The model under review builds one solid part; all positions refer to its coordinate system, in mm. Round coordinates to 2 decimals unless told otherwise and drop trailing zeros. Write each loop counter-clockwise with the first axis right and the second up, starting at its lowest first coordinate (ties: lowest second). Pieces come first, ordered by that corner, then holes. Notation, with made-up numbers: M 52,61.25 L 68,61.25 A35 ccw 68,96.25 Z; hole C 6.5,-38.5 d9. An arc over 180 degrees is marked long. Write item = value, one per line. Start each with the question number.
Item 1: Take a section at C-C, the plane z = -91. Give the boundary of the cut face in (x, y), plus the area to 3 significant figures.
Item 2: For pin 1 Ø1 at (y, z) = (15, -35) entering from -X; pin 2 Ø3 at (x, z) = (105.5, -212.5) entering from +Y; pin 3 Ø5 at (x, z) = (221.5, -97.5) entering from +Y, all flat-tipped, find the tip position at first contact; note any pin that passes through.
Item 3: To check wall thickness, follow line 1 along X through (y, z) = (2.25, -290); line 2 along Z through (x, y) = (260, 0.6); line 3 along X through (y, z) = (2.1, -190). State the ranges of each line that lie inside material, in increasing order.
Item 4: Take a section at A-A, the plane y = 23.5. Give the boundary of the cut face in (x, z), plus the area to 3 significant figures.
Item 5: Take a section at B-B, the plane x = 82. Give the boundary of the cut face in (y, z), plus the area to 3 significant figures.
from build123d import *

# Parameters (mm, degrees)
SKETCH1_W            = 270
SKETCH1_H            = 300
SKETCH1_R            = 2
BOSS_EXTRUDE1_DEPTH  = 3
SKETCH2_R            = 1.35
BOSS_EXTRUDE2_DEPTH  = 10
SKETCH3_R            = 2
BOSS_EXTRUDE3_DEPTH  = 15
SKETCH4_R            = 1.35
BOSS_EXTRUDE4_DEPTH  = 5
SKETCH5_R            = 2
BOSS_EXTRUDE5_DEPTH  = 15
SKETCH6_R            = 1.6
BOSS_EXTRUDE6_DEPTH  = 15
SKETCH7_R            = 2
BOSS_EXTRUDE7_DEPTH  = 15
CUT_EXTRUDE1_START   = -15
SKETCH8_R            = 1.6
CUT_EXTRUDE1_DEPTH   = 15
SKETCH9_R            = 1.6
BOSS_EXTRUDE8_DEPTH  = 15
CUT_EXTRUDE3_START   = -15
SKETCH10_R           = 1.6
CUT_EXTRUDE3_DEPTH   = 15
SKETCH11_R           = 1.6
BOSS_EXTRUDE9_DEPTH  = 15
SKETCH12_R           = 1.6
BOSS_EXTRUDE10_DEPTH = 15
CUT_EXTRUDE4_START   = -15
SKETCH13_R           = 2
CUT_EXTRUDE4_DEPTH   = 15
SKETCH14_R           = 1.35
BOSS_EXTRUDE11_DEPTH = 15
CUT_EXTRUDE7_START   = -15
SKETCH15_R           = 1.35
CUT_EXTRUDE7_DEPTH   = 15
SKETCH16_R           = 1.35
BOSS_EXTRUDE12_DEPTH = 15
SKETCH18_R           = 1.35
CUT_EXTRUDE9_DEPTH   = 15


with BuildPart() as part:
    # Sketch1 → Boss-Extrude1 (new body)
    with BuildSketch(Plane(origin=(0, 0, 0), x_dir=(1, 0, 0), z_dir=(0, 1, 0))):
        with Locations((135, 150)):
            Rectangle(SKETCH1_W, SKETCH1_H)
        with Locations(Location((10, 290, 0), (0, 0, 270))):
            Circle(SKETCH1_R, mode=Mode.SUBTRACT)
        with Locations(Location((10, 190, 0), (0, 0, 270))):
            Circle(SKETCH1_R, mode=Mode.SUBTRACT)
        with Locations(Location((10, 10, 0), (0, 0, 270))):
            Circle(SKETCH1_R, mode=Mode.SUBTRACT)
        with Locations(Location((135, 10, 0), (0, 0, 270))):
            Circle(SKETCH1_R, mode=Mode.SUBTRACT)
        with Locations(Location((260, 290, 0), (0, 0, 90))):
            Circle(SKETCH1_R, mode=Mode.SUBTRACT)
        with Locations(Location((260, 190, 0), (0, 0, 90))):
            Circle(SKETCH1_R, mode=Mode.SUBTRACT)
        with Locations(Location((260, 10, 0), (0, 0, 90))):
            Circle(SKETCH1_R, mode=Mode.SUBTRACT)
        with Locations(Location((135, 290, 0), (0, 0, 270))):
            Circle(SKETCH1_R, mode=Mode.SUBTRACT)
    extrude(amount=BOSS_EXTRUDE1_DEPTH)

    # Sketch2 → Boss-Extrude2 (add)
    with BuildSketch(Plane(origin=(0, 3, 0), x_dir=(1, 0, 0), z_dir=(0, 1, 0))):
        with Locations(Location((106, 270, 0), (0, 0, 90))):
            Circle(SKETCH2_R)
        with Locations(Location((155, 270, 0), (0, 0, 90))):
            Circle(SKETCH2_R)
        with Locations(Location((106, 212, 0), (0, 0, 90))):
            Circle(SKETCH2_R)
        with Locations(Location((155, 212, 0), (0, 0, 90))):
            Circle(SKETCH2_R)
    extrude(amount=BOSS_EXTRUDE2_DEPTH)

    # Sketch3 → Boss-Extrude3 (add)
    with BuildSketch(Plane(origin=(0, 3, 0), x_dir=(1, 0, 0), z_dir=(0, 1, 0))):
        with Locations(Location((150, 172.75, 0), (0, 0, 90))):
            Circle(SKETCH3_R)
        with Locations(Location((150, 127.25, 0), (0, 0, 90))):
            Circle(SKETCH3_R)
    extrude(amount=BOSS_EXTRUDE3_DEPTH)

    # Sketch4 → Boss-Extrude4 (add)
    with BuildSketch(Plane(origin=(0, 13, 0), x_dir=(1, 0, 0), z_dir=(0, 1, 0))):
        with Locations(Location((106, 212, 0), (0, 0, 90))):
            Circle(SKETCH4_R)
        with Locations(Location((155, 212, 0), (0, 0, 90))):
            Circle(SKETCH4_R)
        with Locations(Location((155, 270, 0), (0, 0, 90))):
            Circle(SKETCH4_R)
        with Locations(Location((106, 270, 0), (0, 0, 90))):
            Circle(SKETCH4_R)
    extrude(amount=BOSS_EXTRUDE4_DEPTH)

    # Sketch5 → Boss-Extrude5 (add)
    with BuildSketch(Plane(origin=(0, 3, 0), x_dir=(1, 0, 0), z_dir=(0, 1, 0))):
        with Locations(Location((41, 270, 0), (0, 0, 90))):
            Circle(SKETCH5_R)
        with Locations(Location((71, 270, 0), (0, 0, 90))):
            Circle(SKETCH5_R)
    extrude(amount=BOSS_EXTRUDE5_DEPTH)

    # Sketch6 → Boss-Extrude6 (add)
    with BuildSketch(Plane(origin=(0, 3, 0), x_dir=(1, 0, 0), z_dir=(0, 1, 0))):
        with Locations(Location((65, 75.462075724, 0), (0, 0, 90))):
            Circle(SKETCH6_R)
        with Locations(Location((105, 75.462075724, 0), (0, 0, 90))):
            Circle(SKETCH6_R)
        with Locations(Location((65, 35.462075724, 0), (0, 0, 90))):
            Circle(SKETCH6_R)
        with Locations(Location((105, 35.462075724, 0), (0, 0, 90))):
            Circle(SKETCH6_R)
        with Locations(Location((165, 35.462075724, 0), (0, 0, 90))):
            Circle(SKETCH6_R)
        with Locations(Location((205, 35.462075724, 0), (0, 0, 90))):
            Circle(SKETCH6_R)
        with Locations(Location((205, 75.462075724, 0), (0, 0, 90))):
            Circle(SKETCH6_R)
        with Locations(Location((165, 75.462075724, 0), (0, 0, 90))):
            Circle(SKETCH6_R)
    extrude(amount=BOSS_EXTRUDE6_DEPTH)

    # Sketch7 → Boss-Extrude7 (add)
    with BuildSketch(Plane(origin=(0, 3, 0), x_dir=(1, 0, 0), z_dir=(0, 1, 0))):
        with Locations(Location((41, 230, 0), (0, 0, 90))):
            Circle(SKETCH7_R)
        with Locations(Location((71, 230, 0), (0, 0, 90))):
            Circle(SKETCH7_R)
    extrude(amount=BOSS_EXTRUDE7_DEPTH)

    # Sketch8 → Cut-Extrude1 (cut)
    with BuildSketch(Plane(origin=(0, 18, 0), x_dir=(1, 0, 0), z_dir=(0, 1, 0)).offset(CUT_EXTRUDE1_START)):
        with Locations((205, 75.462075724)):
            Circle(SKETCH8_R)
        with Locations((205, 35.462075724)):
            Circle(SKETCH8_R)
    extrude(amount=CUT_EXTRUDE1_DEPTH, mode=Mode.SUBTRACT)

    # Sketch9 → Boss-Extrude8 (add)
    with BuildSketch(Plane(origin=(0, 3, 0), x_dir=(1, 0, 0), z_dir=(0, 1, 0))):
        with Locations(Location((185, 75.462075724, 0), (0, 0, 90))):
            Circle(SKETCH9_R)
        with Locations(Location((185, 35.462075724, 0), (0, 0, 90))):
            Circle(SKETCH9_R)
    extrude(amount=BOSS_EXTRUDE8_DEPTH)

    # Sketch10 → Cut-Extrude3 (cut)
    with BuildSketch(Plane(origin=(0, 18, 0), x_dir=(1, 0, 0), z_dir=(0, 1, 0)).offset(CUT_EXTRUDE3_START)):
        with Locations((185, 75.462075724)):
            Circle(SKETCH10_R)
        with Locations((185, 35.462075724)):
            Circle(SKETCH10_R)
    extrude(amount=CUT_EXTRUDE3_DEPTH, mode=Mode.SUBTRACT)

    # Sketch11 → Boss-Extrude9 (add)
    with BuildSketch(Plane(origin=(0, 18, 0), x_dir=(1, 0, 0), z_dir=(0, 1, 0))):
        with Locations(Location((205, 75.462075724, 0), (0, 0, 270))):
            Circle(SKETCH11_R)
        with Locations(Location((205, 35.462075724, 0), (0, 0, 270))):
            Circle(SKETCH11_R)
    extrude(amount=-BOSS_EXTRUDE9_DEPTH)

    # Sketch12 → Boss-Extrude10 (add)
    with BuildSketch(Plane(origin=(0, 18, 0), x_dir=(1, 0, 0), z_dir=(0, 1, 0))):
        with Locations(Location((65, 35.462075724, 0), (0, 0, 90))):
            Circle(SKETCH12_R)
        with Locations(Location((105, 35.462075724, 0), (0, 0, 90))):
            Circle(SKETCH12_R)
        with Locations(Location((105, 75.462075724, 0), (0, 0, 90))):
            Circle(SKETCH12_R)
        with Locations(Location((65, 75.462075724, 0), (0, 0, 90))):
            Circle(SKETCH12_R)
        with Locations(Location((165, 75.462075724, 0), (0, 0, 90))):
            Circle(SKETCH12_R)
        with Locations(Location((165, 35.462075724, 0), (0, 0, 90))):
            Circle(SKETCH12_R)
        with Locations(Location((205, 35.462075724, 0), (0, 0, 270))):
            Circle(SKETCH12_R)
        with Locations(Location((205, 75.462075724, 0), (0, 0, 270))):
            Circle(SKETCH12_R)
    extrude(amount=BOSS_EXTRUDE10_DEPTH)

    # Sketch13 → Cut-Extrude4 (cut)
    with BuildSketch(Plane(origin=(0, 18, 0), x_dir=(1, 0, 0), z_dir=(0, 1, 0)).offset(CUT_EXTRUDE4_START)):
        with Locations((41, 270)):
            Circle(SKETCH13_R)
        with Locations((41, 230)):
            Circle(SKETCH13_R)
    extrude(amount=CUT_EXTRUDE4_DEPTH, mode=Mode.SUBTRACT)

    # Sketch14 → Boss-Extrude11 (add)
    with BuildSketch(Plane(origin=(0, 18, 0), x_dir=(1, 0, 0), z_dir=(0, 1, 0))):
        with Locations(Location((155, 190, 0), (0, 0, 270))):
            Circle(SKETCH14_R)
        with Locations(Location((106, 190, 0), (0, 0, 270))):
            Circle(SKETCH14_R)
        with Locations(Location((106, 248, 0), (0, 0, 270))):
            Circle(SKETCH14_R)
        with Locations(Location((155, 248, 0), (0, 0, 90))):
            Circle(SKETCH14_R)
    extrude(amount=-BOSS_EXTRUDE11_DEPTH)

    # Sketch15 → Cut-Extrude7 (cut)
    with BuildSketch(Plane(origin=(0, 18, 0), x_dir=(1, 0, 0), z_dir=(0, 1, 0)).offset(CUT_EXTRUDE7_START)):
        with Locations((106, 212)):
            Circle(SKETCH15_R)
        with Locations((155, 212)):
            Circle(SKETCH15_R)
        with Locations((155, 270)):
            Circle(SKETCH15_R)
        with Locations((106, 270)):
            Circle(SKETCH15_R)
    extrude(amount=CUT_EXTRUDE7_DEPTH, mode=Mode.SUBTRACT)

    # Sketch16 → Boss-Extrude12 (add)
    with BuildSketch(Plane(origin=(0, 18, 0), x_dir=(1, 0, 0), z_dir=(0, 1, 0))):
        with Locations(Location((106, 270, 0), (0, 0, 270))):
            Circle(SKETCH16_R)
        with Locations(Location((155, 270, 0), (0, 0, 270))):
            Circle(SKETCH16_R)
        with Locations(Location((106, 212, 0), (0, 0, 270))):
            Circle(SKETCH16_R)
        with Locations(Location((155, 212, 0), (0, 0, 270))):
            Circle(SKETCH16_R)
    extrude(amount=-BOSS_EXTRUDE12_DEPTH)

    # Sketch18 → Cut-Extrude9 (cut)
    with BuildSketch(Plane(origin=(0, 18, 0), x_dir=(1, 0, 0), z_dir=(0, 1, 0))):
        with Locations((106, 248)):
            Circle(SKETCH18_R)
        with Locations((155, 248)):
            Circle(SKETCH18_R)
        with Locations((155, 190)):
            Circle(SKETCH18_R)
        with Locations((106, 190)):
            Circle(SKETCH18_R)
    extrude(amount=-CUT_EXTRUDE9_DEPTH, mode=Mode.SUBTRACT)


solid = part.part
Response values:
q1.outline = M 0,0 L 270,0 L 270,3 L 0,3 Z
q1.area = 810 mm2
q2.pin_1 = 63.4
q2.pin_2 = 18
q2.pin_3 = 3
q3.line_1 = 0 to 8, 12 to 133, 137 to 258, 262 to 270
q3.line_2 = -300 to -292, -288 to -192, -188 to -12, -8 to 0
q3.line_3 = 0 to 8, 12 to 258, 262 to 270
q4.outline = C 65,-75.46 d3.2; C 65,-35.46 d3.2; C 105,-75.46 d3.2; C 105,-35.46 d3.2; C 165,-75.46 d3.2; C 165,-35.46 d3.2; C 205,-75.46 d3.2; C 205,-35.46 d3.2
q4.area = 64.3 mm2
q5.outline = M 0,-300 L 3,-300 L 3,0 L 0,0 Z
q5.area = 900 mm2
